Geometry: final body of the model. Coordinates: model frame, mm. Face numbers are marked on the shaded views. A direction names the side the tool comes from. Round coordinates to 2 decimals unless told otherwise and drop trailing zeros. Write each loop counter-clockwise with the first axis right and the second up, starting at its lowest first coordinate (ties: lowest second). Pieces come first, ordered by that corner, then holes. Notation, with made-up numbers: (-17, -27) -> (-12, -27) arc R14 cw to (-12, -8) -> close; hole circle Ø1 at (62, 48.5). An arc over 180 degrees is marked (long way). One line per item, written item: value. Start each with the question number.
from build123d import *

# Parameters (mm, degrees)
F0_W      = 80.01
F0_H      = 80.01
F0_W_2    = 69.85
F0_H_2    = 69.85
F1_DEPTH  = 35.56
F2_T      = -2.54
F3_W      = 34.29
F3_H      = 34.29
F3_W_2    = 24.13
F3_H_2    = 24.13
F4_DEPTH  = 25.4
F5_DEPTH  = 30.48
F6_R      = 6.35
F10_DEPTH = 5.08
F7_R      = 6.35
F11_DEPTH = 5.08
F9_R      = 6.35
F12_DEPTH = 5.08
F8_R      = 6.35
F13_DEPTH = 5.08


with BuildPart() as f1:
    # F0 (on Top) → F1 (new body)
    with BuildSketch(Plane.XY):
        with Locations((-40.005, 40.005)):
            Rectangle(F0_W, F0_H)
        with Locations((-40.005, 40.005)):
            Rectangle(F0_W_2, F0_H_2, mode=Mode.SUBTRACT)
        with Locations((-40.005, 40.005)):
            Rectangle(F0_W_2, F0_H_2)
    extrude(amount=F1_DEPTH)

    # F2
    f2_openings = [f1.faces().sort_by_distance(p)[0] for p in [
        (-40.005, 40.005, 35.56),
    ]]
    offset(amount=F2_T, openings=f2_openings)

    # F3 (on face) → F4 (join)
    with BuildSketch(Plane.XY.offset(2.54)):
        with Locations((-40.005, 40.005)):
            Rectangle(F3_W, F3_H)
        with Locations((-40.005, 40.005)):
            Rectangle(F3_W_2, F3_H_2, mode=Mode.SUBTRACT)
    extrude(amount=F4_DEPTH)

    # F5 (add): a face of the model
    f5_faces = [f1.faces().sort_by_distance(p)[0] for p in [
        (-40.005, 40.005, 2.54),
    ]]
    extrude(f5_faces, amount=F5_DEPTH)

    # F6 (on face) → F10 (join)
    with BuildSketch(Plane.XZ.offset(-77.47)):
        with Locations((-12.7, 17.78)):
            Circle(F6_R)
        with Locations((-29.21, 17.78)):
            Circle(F6_R)
        with Locations((-50.8, 17.78)):
            Circle(F6_R)
        with Locations((-67.31, 17.78)):
            Circle(F6_R)
    extrude(amount=F10_DEPTH)

    # F7 (on face) → F11 (join)
    with BuildSketch(Plane(origin=(-2.54, 0, 0), x_dir=(0, -1, 0), z_dir=(-1, 0, 0))):
        with Locations((-12.7, 17.78)):
            Circle(F7_R)
        with Locations((-29.21, 17.78)):
            Circle(F7_R)
        with Locations((-50.8, 17.78)):
            Circle(F7_R)
        with Locations((-67.31, 17.78)):
            Circle(F7_R)
    extrude(amount=F11_DEPTH)

    # F9 (on face) → F12 (join)
    with BuildSketch(Plane.YZ.offset(-77.47)):
        with Locations((67.31, 17.78)):
            Circle(F9_R)
        with Locations((50.8, 17.78)):
            Circle(F9_R)
        with Locations((29.21, 17.78)):
            Circle(F9_R)
        with Locations((12.7, 17.78)):
            Circle(F9_R)
    extrude(amount=F12_DEPTH)

    # F8 (on face) → F13 (join)
    with BuildSketch(Plane(origin=(0, 2.54, 0), x_dir=(-1, 0, 0), z_dir=(0, 1, 0))):
        with Locations((29.21, 17.78)):
            Circle(F8_R)
        with Locations((50.8, 17.78)):
            Circle(F8_R)
        with Locations((67.31, 17.78)):
            Circle(F8_R)
        with Locations((12.7, 17.78)):
            Circle(F8_R)
    extrude(amount=F13_DEPTH)


solid = f1.part
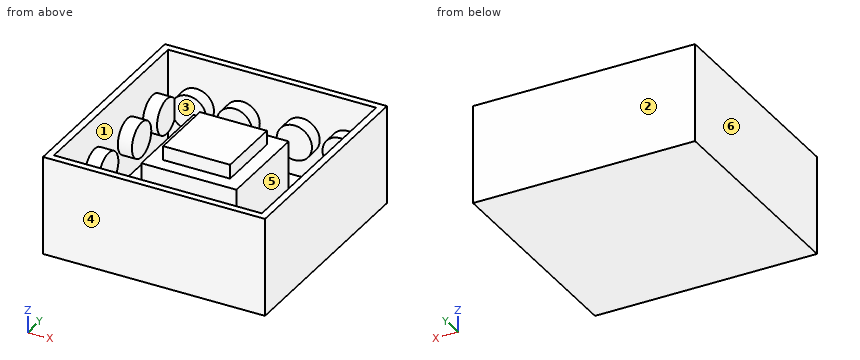
(1) Section query D-D (z = 10). Output: boundary loops of the cut face in (x, y).
(2) Section query B-B (y = 67.31). Output: boundary loops of the cut face in (x, z).
(3) Section query A-A (z = 29). Output: boundary loops of the cut face in (x, y), and give its area (3 significant figures).
(4) Section query C-C (x = -12.7). Output: boundary loops of the cut face in (y, z).
(5) Pull-direction query (X, two-part tool) for the marked faces 4, 5 and 6; classes: pulls with the +X half, pulls with the -X half, needs draft (parallel to the pull), parting line crosses it, or undercut.
(6) Set-up query: the marked faces 1, 2 and 3. Return all of +Z, -Z, +X, -X, +Y, -Y with unobstructed straight access to the full face (end or side cutting, diameter ignored); none if empty.
(7) Line query: probe 1 along Y at (x, z) = (-57, 5.5); probe 2 along X at (y, z) = (32.5, 22); probe 3 along Y at (x, z) = (-50, 32). Output: solid intervals per line, ascending.
(8) Pin query (flat end, axial travel): pin 1 (22.5 mm diameter, centred on x = -46, y = 29, fed in from +Z); pin 2 (2 mm diameter, centred on x = -19.5, y = 21, fed in from +Z). Return the tip coordinate at first contact, or that it passes through.
Results list:
1. outline: (-80.01, 0) -> (0, 0) -> (0, 80.01) -> (-80.01, 80.01) -> close; (-57.15, 22.86) -> (-22.86, 22.86) -> (-22.86, 57.15) -> (-57.15, 57.15) -> close; hole (-77.47, 2.54) -> (-2.54, 2.54) -> (-2.54, 77.47) -> (-77.47, 77.47) -> close
2. outline: (-80.01, 0) -> (0, 0) -> (0, 35.56) -> (-2.54, 35.56) -> (-2.54, 24.13) -> (-7.62, 24.13) -> (-7.62, 11.43) -> (-2.54, 11.43) -> (-2.54, 2.54) -> (-77.47, 2.54) -> (-77.47, 11.43) -> (-72.39, 11.43) -> (-72.39, 24.13) -> (-77.47, 24.13) -> (-77.47, 35.56) -> (-80.01, 35.56) -> close
3. outline: (-80.01, 0) -> (0, 0) -> (0, 80.01) -> (-80.01, 80.01) -> close; (-52.07, 27.94) -> (-27.94, 27.94) -> (-27.94, 52.07) -> (-52.07, 52.07) -> close; hole (-77.47, 2.54) -> (-2.54, 2.54) -> (-2.54, 77.47) -> (-77.47, 77.47) -> close
3. area: 1,370 mm^2
4. outline: (0, 0) -> (80.01, 0) -> (80.01, 35.56) -> (77.47, 35.56) -> (77.47, 24.13) -> (72.39, 24.13) -> (72.39, 11.43) -> (77.47, 11.43) -> (77.47, 2.54) -> (2.54, 2.54) -> (2.54, 11.43) -> (7.62, 11.43) -> (7.62, 24.13) -> (2.54, 24.13) -> (2.54, 35.56) -> (0, 35.56) -> close
5. face 4: needs draft
5. face 5: undercut
5. face 6: pulls with the -X half
6. face 1: none
6. face 2: +Z, -Z, +X, -X, +Y
6. face 3: +Z
7. probe 1: y = 0 to 2.54, 22.86 to 57.15, 77.47 to 80.01
7. probe 2: x = -80.01 to -72.39, -57.15 to -22.86, -7.62 to 0
7. probe 3: y = 0 to 2.54, 27.94 to 52.07, 77.47 to 80.01
8. pin 1: stops at z = 33.02
8. pin 2: stops at z = 2.54
